Autodesk Inventor part; units mm, degrees
ref_plane "YZ Plane" through (0, 0, 0) normal (1, 0, 0) x (0, 1, 0)
ref_plane "XZ Plane" through (0, 0, 0) normal (0, 1, 0) x (-1, 0, 0)
ref_plane "XY Plane" through (0, 0, 0) normal (0, 0, 1) x (1, 0, 0)
sketch "Sketch1" plane through (0, 0, 0) normal (0, 0, 1) x (1, 0, 0)
  circle A0 centre (0, 0) radius 6.35
  line L0 (-6.35, 0) -> (-6.35, 12.7)
  line L1 (-6.35, 12.7) -> (6.35, 12.7)
  line L2 (6.35, 12.7) -> (6.35, 0)
  dimension "d0" = 12.7
  dimension "d1" = 12.7
extrude "Extrusion1" add sketch "Sketch1" along normal blind 6.35
hole "Hole1" at (0, 0, 0) direction (0, 0, 1) diameter 5.1054 end through all
sketch "Sketch2" plane through (-6.35, 12.7, 0) normal (0, 1, 0) x (1, 0, 0)
  line L0 (6.35, 0) -> (19.05, 0) construction
  line L1 (6.35, 0) -> (-6.35, 0) construction
  line L2 (-6.35, 0) -> (6.35, 21.997) construction
  line L3 (6.35, 21.997) -> (19.05, 0) construction
  circle A0 centre (19.05, 0) radius 6.35 construction
  circle A1 centre (-6.35, 0) radius 6.35 construction
  circle A2 centre (6.35, 21.997) radius 6.35 construction
  line L4 (0.8507, 25.172) -> (-11.8493, 3.175)
  line L5 (11.8493, 25.172) -> (24.5493, 3.175)
  line L6 (19.05, -6.35) -> (12.7, -6.35)
  line L7 (0, -6.35) -> (12.7, -6.35)
  line L8 (12.7, -6.35) -> (0, -6.35)
  line L9 (0, -6.35) -> (-6.35, -6.35)
  arc A3 (-11.8493, 3.175) -> (-6.35, -6.35) centre (-6.35, 0) ccw
  arc A4 (11.8493, 25.172) -> (0.8507, 25.172) centre (6.35, 21.997) ccw
  arc A5 (19.05, -6.35) -> (24.5493, 3.175) centre (19.05, 0) ccw
  dimension "d11" = 12.7
  dimension "d12" = 12.7
  dimension "d13" = 25.4
  dimension "d14" = 25.4
  dimension "d15" = 12.7
  dimension "d16" = 12.7
  dimension "d17" = 12.7
extrude "Extrusion2" add sketch "Sketch2" along normal blind 3.175
hole "Hole2" at (12.7, 12.7, 0) at (0, 12.7, -21.997) at (-12.7, 12.7, 0) direction (0, 1, 0) diameter 5.1054 end through all
properties part number "Table Holder"
Part model, mm, in its own coordinate system. A direction names the side the tool comes from. Coordinates: 2 decimals unless noted, no trailing zeros. Loops run counter-clockwise (first coordinate to the right, second up) from the corner with the lowest first, then second, coordinate; pieces in that order, holes last. Notation, with made-up numbers: (83.25, 18) - (91.25, 18) arc R23 ccw to (91.25, 57) - close; hole circle Ø6 at (5, 21). An arc over 180 degrees is marked (long way). Write each question's results on one line, items separated by ' | '. Start each with the question number.
Q1. Slice it at D-D on y = 0.5. Give the cut face in (x, z), and give its area (3 significant figures).
Q2. Two-plate mould, pull along X, no slides. Class faces 1 (the cylindrical face through (0.14, -6.35, 3.13)), 2 (the flat face through (0, 12.7, -7)), 3 (the cylindrical face through (-10.208, 14.31, 0.553)): +X half, -X half, draft (parallel to the pull), parting line (faces both ways), or undercut.
Q3. Probe line 1 along X through (y, z) = (15.1, 0); line 2 along Y through (x, z) = (0, 1.75) (3 decimals); line 3 along Z through (x, y) = (12.7, 13.95). List the from-to ranges inside material, lowest first.
Q4. Slice it at B-B on y = 13.25. Give the cut face in (x, z) (3 decimals), and give its area (3 significant figures).
Q5. Drop flat-ended pins along their axis: pin 1 Ø6 at (x, y) = (0.5, -1.5) entering from +Z; pin 2 Ø5 at (x, z) = (6, -3) entering from -Y; pin 3 Ø3 at (y, z) = (3.5, 2.5) entering from -X; pin 4 Ø3 at (y, z) = (9, 2.5) entering from +X. Give the stop position or say it passes through.
Q6. Slice it at A-A on x = 0. Give the cut face in (y, z) (3 decimals), and give its area (3 significant figures).
Q7. Which spindle directions (+Z, -Z, +X, -X, +Y, -Y) get a long thin tool onto all of the face, cutting with end or side? Do faces 4 (the flat face through (6.35, 6, 3)), 5 (the flat face through (0, 7, 6.35)), 6 (the flat face through (-6.35, 6, 3)), 7 (the flat face through (0, 3, 0)), 8 (the cylindrical face through (18.245, 14.265, 3.094)). Say none if no direction does.
Q8. Slice it at C-C on z = -22.5. Give the cut face in (x, y) (3 decimals), and give its area (3 significant figures).
Answer:
1) outline: (-6.35, 0) - (-2.5, 0) - (-2.5, 6.35) - (-6.35, 6.35) - close; (2.5, 0) - (6.35, 0) - (6.35, 6.35) - (2.5, 6.35) - close | area: 48.9 mm2
2) face 1: parting line | face 2: draft | face 3: undercut
3) line 1: x = -19.05 to -15.25, -10.15 to 10.15, 15.25 to 19.05 | line 2: y = -6.35 to -2.553, 2.553 to 15.875 | line 3: z = -12.7 to -2.55, 2.55 to 6.35
4) outline: (-18.199, -3.175) - (-5.499, -25.172) arc R6.35 ccw to (5.499, -25.172) - (18.199, -3.175) arc R6.35 ccw to (12.7, 6.35) - (-12.7, 6.35) arc R6.35 ccw to start; hole circle Ø5.105 at (-12.7, 0); hole circle Ø5.105 at (0, -21.997); hole circle Ø5.105 at (12.7, 0) | area: 828 mm2
5) pin 1: stops at z = 6.35 | pin 2: stops at y = 12.7 | pin 3: stops at x = -6.35 | pin 4: stops at x = 6.35
6) outline: (-6.35, 0) - (-2.553, 0) - (-2.553, 6.35) - (-6.35, 6.35) - close; (2.553, 0) - (12.7, 0) - (12.7, -19.444) - (15.875, -19.444) - (15.875, 6.35) - (2.553, 6.35) - close; (12.7, -28.347) - (15.875, -28.347) - (15.875, -24.55) - (12.7, -24.55) - close | area: 183 mm2
7) face 4: +Z, -Z, +X, -Y | face 5: +Z, +X, -X, +Y, -Y | face 6: +Z, -Z, -X, -Y | face 7: -Z, +X, -X, -Y | face 8: +X, +Y, -Y
8) outline: (-7.042, 12.7) - (-2.503, 12.7) - (-2.503, 15.875) - (-7.042, 15.875) - close; (2.503, 12.7) - (7.042, 12.7) - (7.042, 15.875) - (2.503, 15.875) - close | area: 28.8 mm2
